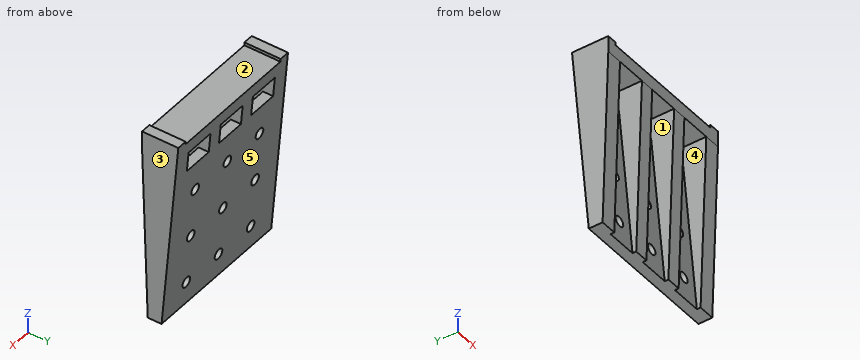
from build123d import *

# Parameters (mm, degrees)
F0_W      = 75
F0_H      = 100
F1_DEPTH  = 18
F3_DEPTH  = 75.001
F4_W      = 15
F4_H      = 92
F5_DEPTH  = 50
F6_W      = 65
F6_H      = 18
F7_DEPTH  = 1.5
F9_DEPTH  = 75.001
F11_DEPTH = 75
F12_W     = 65
F12_H     = 1.5
F13_DEPTH = 18.001
F14_W     = 15
F14_H     = 10
F14_W_2   = 75.273126
F14_H_2   = 5
F14_R     = 2.6
F15_DEPTH = 18.001


with BuildPart() as f1:
    # F0 (on Front) → F1 (new body)
    with BuildSketch(Plane.XZ):
        with Locations((37.5, 50)):
            Rectangle(F0_W, F0_H)
    extrude(amount=F1_DEPTH)

    # F2 (on face) → F3 (cut, through all)
    with BuildSketch(Plane(origin=(0, 0, 0), x_dir=(0, -1, 0), z_dir=(-1, 0, 0))):
        Polygon((18, 92), (15, 0), (18, 0), align=None)
    extrude(amount=-F3_DEPTH, mode=Mode.SUBTRACT)

    # F4 (on face) → F5 (cut)
    with BuildSketch(Plane.XZ.offset(18)):
        with Locations((15.5, 46)):
            Rectangle(F4_W, F4_H)
        with Locations((37.5, 46)):
            Rectangle(F4_W, F4_H)
        with Locations((59.5, 46)):
            Rectangle(F4_W, F4_H)
    extrude(amount=-F5_DEPTH, mode=Mode.SUBTRACT)

    # F6 (on face) → F7 (cut)
    with BuildSketch(Plane.XY.offset(100)):
        with Locations((37.5, -9)):
            Rectangle(F6_W, F6_H)
    extrude(amount=-F7_DEPTH, mode=Mode.SUBTRACT)

    # F8 (on face) → F9 (cut, through all)
    with BuildSketch(Plane(origin=(0, 0, 0), x_dir=(0, -1, 0), z_dir=(-1, 0, 0))):
        Polygon((8.748866, 0), (0, 100), (0, 0), align=None)
    extrude(amount=-F9_DEPTH, mode=Mode.SUBTRACT)

    # F10 (on face) → F11 (join, through all)
    with BuildSketch(Plane(origin=(0, 0, 0), x_dir=(0, -1, 0), z_dir=(-1, 0, 0))):
        Polygon((5.019099, 100), (0, 100), (8.748866, 0), (13.767966, 0), align=None)
    extrude(amount=-F11_DEPTH)

    # F12 (on face) → F13 (cut, through all)
    with BuildSketch(Plane.XZ.offset(18)):
        with Locations((37.5, 99.25)):
            Rectangle(F12_W, F12_H)
    extrude(amount=-F13_DEPTH, mode=Mode.SUBTRACT)

    # F14 (on face) → F15 (cut, through all)
    with BuildSketch(Plane.XZ.offset(18)):
        with Locations((15.5, 87)):
            Rectangle(F14_W, F14_H)
        with Locations((37.5, 87)):
            Rectangle(F14_W, F14_H)
        with Locations((59.5, 87)):
            Rectangle(F14_W, F14_H)
        with Locations((37.636563, 2.5)):
            Rectangle(F14_W_2, F14_H_2)
        with Locations((15.5, 67)):
            Circle(F14_R)
        with Locations((37.5, 67)):
            Circle(F14_R)
        with Locations((59.5, 67)):
            Circle(F14_R)
        with Locations((59.5, 42)):
            Circle(F14_R)
        with Locations((37.5, 42)):
            Circle(F14_R)
        with Locations((37.5, 17)):
            Circle(F14_R)
        with Locations((59.5, 17)):
            Circle(F14_R)
        with Locations((15.5, 17)):
            Circle(F14_R)
        with Locations((15.5, 42)):
            Circle(F14_R)
    extrude(amount=-F15_DEPTH, mode=Mode.SUBTRACT)


solid = f1.part
Geometry: final body of the model. Coordinates: model frame, mm. Face numbers are marked on the shaded views. A direction names the side the tool comes from. Give positions to 0.01 mm unless a question says otherwise; leave off trailing zeros. Write each loop counter-clockwise with the first axis right and the second up, starting at its lowest first coordinate (ties: lowest second). Pieces come first, ordered by that corner, then holes.
(1) Cut plane D-D, the plane z = 86.5. Return loops of the section in (x, y), then the cut area to 3 significant figures.
(2) Cut plane A-A, the plane x = 53.5. Return loops of the section in (y, z), then the cut area to 3 significant figures.
(3) Access query for the marked faces 4 and 5. Directions: +Z, -Z, +X, -X, +Y, -Y. A direction counts if a zero-diameter tool reaches every point of the face in a straight line with its end or side. Return the directions, or none.
(4) First-contact query: P1, Ø8, axis at x = 26, z = 88.5, coming from the +Y side; P2, Ø2.5, axis at x = 35.5, y = -3.5, coming from the +Z side; P3, Ø1.5, axis at x = 31, z = 19, coming from the +Y side. Flat tips, straight axial feed; report the tip coordinate or a pass-through.
(5) Ray query, line 1 (X direction, y = -10.8, z = 17); line 2 (X direction, y = -11.25, z = 63.5); line 3 (Z direction, x = 39, y = -15.25). Return the intervals inside material, ascending.
(6) Mould query, pull axis Z, two halves, no side actions, for the marked faces 1, 2 and 3. Classes: released by +Z, released by -Z, zero draft, split by the parting line, or undercut.
(7) Cut plane B-B, the plane z = 67. Return loops of the section in (x, y).
(8) Cut plane C-C, the plane x = 14. Return loops of the section in (y, z), then the cut area to 3 significant figures.
Values follow:
1. outline: (0, -17.82) - (8, -17.82) - (8, -1.18) - (0, -1.18) - close; (23, -17.82) - (30, -17.82) - (30, -1.18) - (23, -1.18) - close; (45, -17.82) - (52, -17.82) - (52, -1.18) - (45, -1.18) - close; (67, -17.82) - (75, -17.82) - (75, -1.18) - (67, -1.18) - close
1. area: 499 mm2
2. outline: (-18, 92) - (-0.7, 92) - (-0.13, 98.5) - (-18, 98.5) - close; (-13.33, 5) - (-8.31, 5) - (-1.57, 82) - (-6.59, 82) - close
2. area: 501 mm2
3. face 4: -Y
3. face 5: -Z, +X, -X, +Y
4. P1: stops at y = -0.66
4. P2: stops at z = 98.5
4. P3: stops at y = -7.02
5. line 1: x = 0 to 12.9, 18.1 to 34.9, 40.1 to 56.9, 62.1 to 75
5. line 2: x = 0 to 8, 23 to 30, 45 to 52, 67 to 75
5. line 3: z = 92 to 98.5
6. face 1: undercut
6. face 2: released by +Z
6. face 3: zero draft
7. outline: (0, -17.18) - (8, -17.18) - (8, -7.91) - (12.9, -7.91) - (12.9, -2.89) - (0, -2.89) - close; (18.1, -7.91) - (23, -7.91) - (23, -17.18) - (30, -17.18) - (30, -7.91) - (34.9, -7.91) - (34.9, -2.89) - (18.1, -2.89) - close; (40.1, -7.91) - (45, -7.91) - (45, -17.18) - (52, -17.18) - (52, -7.91) - (56.9, -7.91) - (56.9, -2.89) - (40.1, -2.89) - close; (62.1, -7.91) - (67, -7.91) - (67, -17.18) - (75, -17.18) - (75, -2.89) - (62.1, -2.89) - close
8. outline: (-18, 92) - (-0.7, 92) - (-0.13, 98.5) - (-18, 98.5) - close; (-13.33, 5) - (-8.31, 5) - (-7.45, 14.88) - (-12.47, 14.88) - close; (-12.09, 19.12) - (-7.08, 19.12) - (-5.26, 39.88) - (-10.28, 39.88) - close; (-9.91, 44.12) - (-4.89, 44.12) - (-3.07, 64.88) - (-8.09, 64.88) - close; (-7.72, 69.12) - (-2.7, 69.12) - (-1.57, 82) - (-6.59, 82) - close
8. area: 437 mm2
